```python
from build123d import *

# Parameters (mm, degrees)
SKETCH1_W          = 189
SKETCH1_H          = 208
BASE_FLANGE1_DEPTH = 1
EDGE_FLANGE1_DEPTH = 189
EDGE_FLANGE2_DEPTH = 208
EDGE_FLANGE3_DEPTH = 189
EDGE_FLANGE4_DEPTH = 208
SKETCH17_W         = 21
SKETCH17_H         = 60
CUT_EXTRUDE1_DEPTH = 144.472122728
SKETCH18_W         = 80
SKETCH18_H         = 10
CUT_EXTRUDE2_DEPTH = 10
SKETCH20_R         = 1.5
CUT_EXTRUDE3_DEPTH = 10
SKETCH21_R         = 1
CUT_EXTRUDE4_DEPTH = 10
SKETCH22_R         = 1.5
CUT_EXTRUDE5_DEPTH = 10
SKETCH23_W         = 35
SKETCH23_H         = 10
CUT_EXTRUDE6_DEPTH = 10


# Sheet-metal steps are written as plain solids
with BuildPart() as part:
    # Sketch1 → Base-Flange1 (new body)
    with BuildSketch(Plane(origin=(0, 0, 0), x_dir=(1, 0, 0), z_dir=(0, 1, 0))):
        Rectangle(SKETCH1_W, SKETCH1_H)
    extrude(amount=-BASE_FLANGE1_DEPTH)

    # Edge-Flange1 section (across the edge) → Edge-Flange1 (add)
    with BuildSketch(Plane(origin=(94.5, -1, 105), x_dir=(0, 0, -1), z_dir=(-1, 0, 0))):
        with BuildLine():
            Line((-1, 1), (-1, 5))
            Line((-1, 5), (0, 5))
            Line((0, 5), (0, 1))
            ThreePointArc((0, 1), (0.292893219, 0.292893219), (1, 0))
            Line((1, 0), (1, -1))
            ThreePointArc((1, -1), (-0.414213562, -0.414213562), (-1, 1))
        make_face()
    extrude(amount=EDGE_FLANGE1_DEPTH)

    # Edge-Flange2 section (across the edge) → Edge-Flange2 (add)
    with BuildSketch(Plane(origin=(95.5, -1, -104), x_dir=(-1, 0, 0), z_dir=(0, 0, 1))):
        with BuildLine():
            Line((-1, 1), (-1, 5))
            Line((-1, 5), (0, 5))
            Line((0, 5), (0, 1))
            ThreePointArc((0, 1), (0.292893219, 0.292893219), (1, 0))
            Line((1, 0), (1, -1))
            ThreePointArc((1, -1), (-0.414213562, -0.414213562), (-1, 1))
        make_face()
    extrude(amount=EDGE_FLANGE2_DEPTH)

    # Edge-Flange3 section (across the edge) → Edge-Flange3 (add)
    with BuildSketch(Plane(origin=(-94.5, -1, -105), x_dir=(0, 0, 1), z_dir=(1, 0, 0))):
        with BuildLine():
            Line((-1, 1), (-1, 5))
            Line((-1, 5), (0, 5))
            Line((0, 5), (0, 1))
            ThreePointArc((0, 1), (0.292893219, 0.292893219), (1, 0))
            Line((1, 0), (1, -1))
            ThreePointArc((1, -1), (-0.414213562, -0.414213562), (-1, 1))
        make_face()
    extrude(amount=EDGE_FLANGE3_DEPTH)

    # Edge-Flange4 section (across the edge) → Edge-Flange4 (add)
    with BuildSketch(Plane(origin=(-95.5, -1, 104), x_dir=(1, 0, 0), z_dir=(0, 0, -1))):
        with BuildLine():
            Line((-1, 1), (-1, 5))
            Line((-1, 5), (0, 5))
            Line((0, 5), (0, 1))
            ThreePointArc((0, 1), (0.292893219, 0.292893219), (1, 0))
            Line((1, 0), (1, -1))
            ThreePointArc((1, -1), (-0.414213562, -0.414213562), (-1, 1))
        make_face()
    extrude(amount=EDGE_FLANGE4_DEPTH)

    # Sketch17 → Cut-Extrude1 (cut, through all)
    with BuildSketch(Plane(origin=(0, 0, 0), x_dir=(1, 0, 0), z_dir=(0, 1, 0))):
        with Locations((86, -76)):
            Rectangle(SKETCH17_W, SKETCH17_H)
        with Locations((-86, -76)):
            Rectangle(SKETCH17_W, SKETCH17_H)
    extrude(amount=-CUT_EXTRUDE1_DEPTH, mode=Mode.SUBTRACT)

    # Sketch18 → Cut-Extrude2 (cut)
    with BuildSketch(Plane(origin=(0, 0, 0), x_dir=(1, 0, 0), z_dir=(0, 1, 0))):
        with Locations((0, 99)):
            Rectangle(SKETCH18_W, SKETCH18_H)
    extrude(amount=-CUT_EXTRUDE2_DEPTH, mode=Mode.SUBTRACT)

    # Sketch20 → Cut-Extrude3 (cut)
    with BuildSketch(Plane(origin=(0, 0, 0), x_dir=(1, 0, 0), z_dir=(0, 1, 0))):
        with Locations(Location((-79.5844, -27.41485418, 0), (0, 0, 270))):
            Circle(SKETCH20_R)
        with Locations(Location((-12.0844, -22.41485418, 0), (0, 0, 270))):
            Circle(SKETCH20_R)
        with Locations(Location((-12.0844, 5.08514582, 0), (0, 0, 270))):
            Circle(SKETCH20_R)
        with Locations(Location((-79.5844, 10.08514582, 0), (0, 0, 270))):
            Circle(SKETCH20_R)
    extrude(amount=-CUT_EXTRUDE3_DEPTH, mode=Mode.SUBTRACT)

    # Sketch21 → Cut-Extrude4 (cut)
    with BuildSketch(Plane(origin=(0, 0, 0), x_dir=(1, 0, 0), z_dir=(0, 1, 0))):
        with Locations(Location((68.5, 87.449623923, 0), (0, 0, 270))):
            Circle(SKETCH21_R)
        with Locations(Location((86.058283099, 87.449623923, 0), (0, 0, 270))):
            Circle(SKETCH21_R)
        with Locations(Location((68.5, 69.449623923, 0), (0, 0, 270))):
            Circle(SKETCH21_R)
        with Locations(Location((86.058283099, 69.449623923, 0), (0, 0, 270))):
            Circle(SKETCH21_R)
        with Locations(Location((-86.058283099, 87.449623923, 0), (0, 0, 270))):
            Circle(SKETCH21_R)
        with Locations(Location((-86.058283099, 69.449623923, 0), (0, 0, 270))):
            Circle(SKETCH21_R)
        with Locations(Location((-68.5, 69.449623923, 0), (0, 0, 270))):
            Circle(SKETCH21_R)
        with Locations(Location((-68.5, 87.449623923, 0), (0, 0, 270))):
            Circle(SKETCH21_R)
    extrude(amount=-CUT_EXTRUDE4_DEPTH, mode=Mode.SUBTRACT)

    # Sketch22 → Cut-Extrude5 (cut)
    with BuildSketch(Plane(origin=(0, 0, 0), x_dir=(1, 0, 0), z_dir=(0, 1, 0))):
        with Locations(Location((67.5, -55.5, 0), (0, 0, 270))):
            Circle(SKETCH22_R)
        with Locations(Location((34, -55.5, 0), (0, 0, 270))):
            Circle(SKETCH22_R)
        with Locations(Location((34, -94.5, 0), (0, 0, 270))):
            Circle(SKETCH22_R)
        with Locations(Location((67.5, -94.5, 0), (0, 0, 270))):
            Circle(SKETCH22_R)
        with Locations(Location((-67.5, -94.5, 0), (0, 0, 270))):
            Circle(SKETCH22_R)
        with Locations(Location((-34, -94.5, 0), (0, 0, 270))):
            Circle(SKETCH22_R)
        with Locations(Location((-34, -55.5, 0), (0, 0, 270))):
            Circle(SKETCH22_R)
        with Locations(Location((-67.5, -55.5, 0), (0, 0, 270))):
            Circle(SKETCH22_R)
    extrude(amount=-CUT_EXTRUDE5_DEPTH, mode=Mode.SUBTRACT)

    # Sketch23 → Cut-Extrude6 (cut)
    with BuildSketch(Plane(origin=(0, 0, 0), x_dir=(1, 0, 0), z_dir=(0, 1, 0))):
        with Locations((0, 43.4732)):
            Rectangle(SKETCH23_W, SKETCH23_H)
        with Locations((0, -51)):
            Rectangle(SKETCH23_W, SKETCH23_H)
    extrude(amount=-CUT_EXTRUDE6_DEPTH, mode=Mode.SUBTRACT)


solid = part.part
```
Can you work these out from the model? Positions are in its coordinate system, mm. A direction names the side the tool comes from. Coordinates: 2 decimals unless noted, no trailing zeros. Loops run counter-clockwise (first coordinate to the right, second up) from the corner with the lowest first, then second, coordinate; pieces in that order, holes last.
1) Imagine slicing it at C-C on x = -62. List the corners of the cut face in (y, z) for me.
2) For pin 1 (5 mm diameter, centred on x = 34, z = 51.5, fed in from -Y); pin 2 (1 mm diameter, centred on y = -2.5, z = -105, fed in from -X); pin 3 (1.1 mm diameter, centred on y = -0.5, z = 50, fed in from -X), each with a flat end and sliding along its axis, tell me the tip position at first contact or that it passes through.
3) Imagine slicing it at A-A on x = -5.5. List the corners of the cut face in (y, z) for me, plus the area to 3 significant figures.
4) Thinking about a two-plate mould opening in X: for faces 1 (the flat face through (-1, -1, -1)), 2 (the flat face through (-75.5, -0.5, 80.6)), 3 (the flat face through (-87.6, -0.8, 46)), which applies, pulls with the +X half, pulls with the -X half, needs draft (parallel to the pull), parting line crosses it, or undercut?
5) Which directions (+Z, -Z, +X, -X, +Y, -Y) give clear straight access to the entire face, cutting with the end or side of a thin tool? Please do faces 4 (the flat face through (-1, 0, -1)), 5 (the flat face through (75.5, -0.5, 80.6)).
6) I need wall thicknesses on probe 1 along X at (y, z) = (-0.75, 94.5); probe 2 along Z at (x, y) = (51, -3.95); probe 3 along X at (y, z) = (-0.3, 55.5). Which ranges of each line are inside material? Lowest first, please.
7) Imagine slicing it at D-D on z = 66. List the corners of the cut face in (x, y) for me.
8) Imagine slicing it at B-B on z = 38. List the corners of the cut face in (x, y) for me, plus the area to 3 significant figures.
Completed:
1. outline: (-6, -106) - (-2, -106) arc R2 ccw to (0, -104) - (0, 104) arc R2 ccw to (-2, 106) - (-6, 106) - (-6, 105) - (-2, 105) arc R1 cw to (-1, 104) - (-1, -104) arc R1 cw to (-2, -105) - (-6, -105) - close
2. pin 1: stops at y = -1
2. pin 2: stops at x = -94.5
2. pin 3: stops at x = -75.5
3. outline: (-6, -106) - (-2, -106) arc R2 ccw to (0, -104) - (-1, -104) arc R1 cw to (-2, -105) - (-6, -105) - close; (-6, 105) - (-2, 105) arc R1 cw to (-1, 104) - (-1, 56) - (0, 56) - (0, 104) arc R2 ccw to (-2, 106) - (-6, 106) - close; (-1, -94) - (0, -94) - (0, -48.47) - (-1, -48.47) - close; (-1, -38.47) - (0, -38.47) - (0, 46) - (-1, 46) - close
3. area: 191 mm2
4. face 1: undercut
4. face 2: pulls with the -X half
4. face 3: needs draft
5. face 4: +Z, -Z, +X, -X, +Y
5. face 5: +Z, +X, +Y, -Y
6. probe 1: x = -75.5 to -69, -66 to -35.5, -32.5 to 32.5, 35.5 to 66, 69 to 75.5
6. probe 2: z = -106 to -105, 105 to 106
6. probe 3: x = -75.5 to -69, -66 to -35.5, -32.5 to -17.5, 17.5 to 32.5, 35.5 to 66, 69 to 75.5
7. outline: (-75.5, -1) - (75.5, -1) - (75.5, 0) - (-75.5, 0) - close
8. outline: (-96.5, -6) - (-95.5, -6) - (-95.5, -2) arc R1 cw to (-94.5, -1) - (94.5, -1) arc R1 cw to (95.5, -2) - (95.5, -6) - (96.5, -6) - (96.5, -2) arc R2 ccw to (94.5, 0) - (-94.5, 0) arc R2 ccw to (-96.5, -2) - close
8. area: 202 mm2
